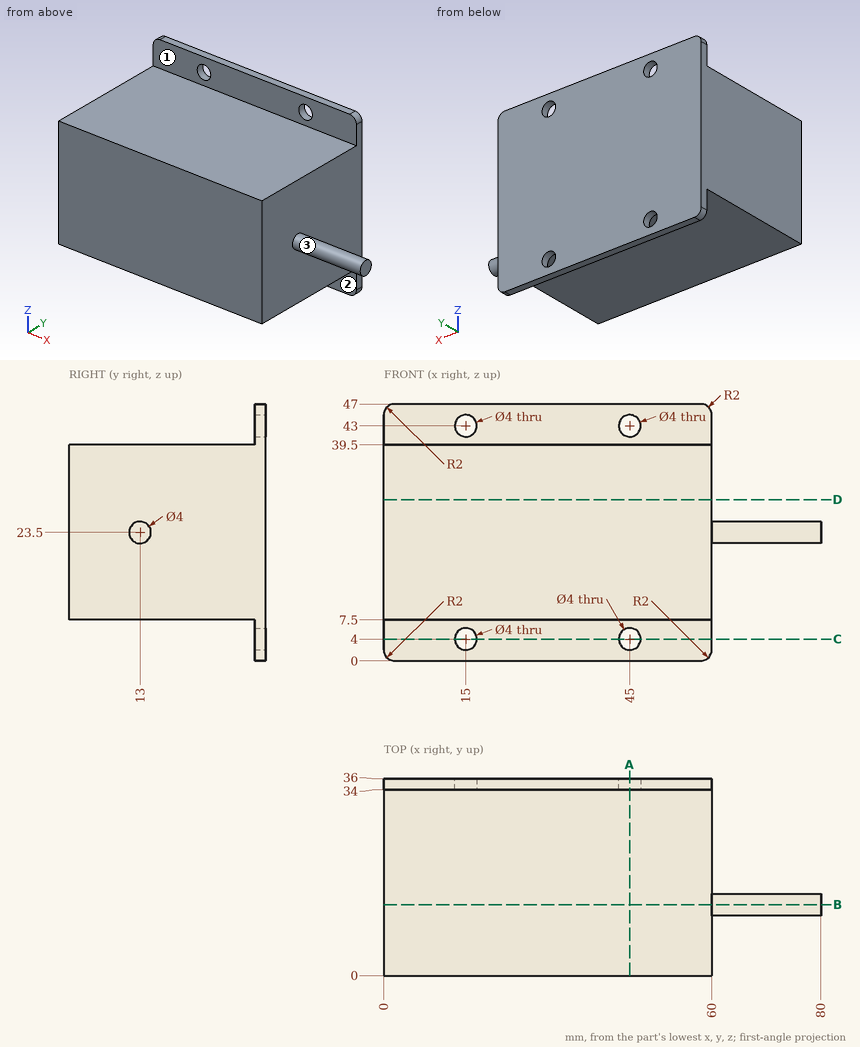
Part print with two shaded views. Sizes in mm from the minimum x, y, z corner. A direction names the side the tool comes from. Give positions to 0.01 mm unless a question says otherwise; leave off trailing zeros. Order: outer loops, then holes, each group sorted by start corner. A loop starts at its lowest first (then second) coordinate and runs counter-clockwise, first axis right, second up.
(1) Flat gauge pins, fed straight in: pin 1 (1.5 mm diameter, centred on x = 59, y = 10.5, fed in from -Z); pin 2 (1.5 mm diameter, centred on x = 39.5, y = 11, fed in from +Z); pin 3 (12 mm diameter, centred on y = 16, z = 13.5, fed in from +X); pin 4 (2.5 mm diameter, centred on x = 45, z = 43, fed in from +Y). Where does each tip first touch, or does it go through?
(2) Saw through at B-B, the plane y = 13. Give the cut face in (x, z), then the cut area to 3 significant figures.
(3) Saw through at C-C, the plane z = 4. Give the cut face in (x, y).
(4) Tool access for the marked faces 1, 2 and 3: list every direction of +Z, -Z, +X, -X, +Y, -Y with a clear straight run to the whole face (end or side of a thin tool).
(5) Saw through at A-A, the plane x = 45. Give the cut face in (y, z), then the cut area to 3 significant figures.
(6) Drill centre lines: L1, parallel to Z at x = 45, y = 35.3; L2, parallel to Z at x = 14.5, y = 9.5; L3, parallel to X at y = 18, z = 26. Where is each one in solid material? Low to high.
(7) Saw through at D-D, the plane z = 29.5. Give the cut face in (x, y), then the cut area to 3 significant figures.
Results found:
1. pin 1: stops at z = 7.5
1. pin 2: stops at z = 39.5
1. pin 3: stops at x = 60
1. pin 4: passes through
2. outline: (0, 7.5) - (60, 7.5) - (60, 21.5) - (80, 21.5) - (80, 25.5) - (60, 25.5) - (60, 39.5) - (0, 39.5) - close
2. area: 2,000 mm2
3. outline: (0, 34) - (13, 34) - (13, 36) - (0, 36) - close; (17, 34) - (43, 34) - (43, 36) - (17, 36) - close; (47, 34) - (60, 34) - (60, 36) - (47, 36) - close
4. face 1: +Z, +X, -X, -Y
4. face 2: -Z, +X, -X, -Y
4. face 3: +X
5. outline: (0, 7.5) - (34, 7.5) - (34, 6) - (36, 6) - (36, 41) - (34, 41) - (34, 39.5) - (0, 39.5) - close; (34, 0) - (36, 0) - (36, 2) - (34, 2) - close; (34, 45) - (36, 45) - (36, 47) - (34, 47) - close
5. area: 1,170 mm2
6. L1: z = 0 to 2, 6 to 41, 45 to 47
6. L2: z = 7.5 to 39.5
6. L3: x = 0 to 60
7. outline: (0, 0) - (60, 0) - (60, 36) - (0, 36) - close
7. area: 2,160 mm2
